```python
from build123d import *

# Parameters (mm, degrees)
ESBO_O1_W                = 4
ESBO_O1_H                = 4
RESSALTO_EXTRUS_O1_DEPTH = 1000
PADR_OCIRCULAR1_COUNT    = 4
FILETE1_R                = 1


with BuildPart() as part:
    # Esboço1 → Ressalto-extrusão1 (new body)
    with BuildSketch(Plane.XY):
        with BuildLine():
            ThreePointArc((-1.664601464, 3.078815026), (-0.858529967, 3.393070335), (0, 3.5))
            Line((0, 3.5), (0, 6))
            Line((0, 6), (-3.878679656, 6))
            Line((-3.878679656, 6), (-8.5, 10.621320344))
            Line((-8.5, 10.621320344), (-8.5, 13))
            Line((-8.5, 13), (-4.1, 13))
            Line((-4.1, 13), (-4.1, 14.5))
            Line((-4.1, 14.5), (-5.1, 14.5))
            Line((-5.1, 14.5), (-5.1, 15))
            Line((-5.1, 15), (-15, 15))
            Line((-15, 15), (-15, 5.1))
            Line((-15, 5.1), (-14.5, 5.1))
            Line((-14.5, 5.1), (-14.5, 4.1))
            Line((-14.5, 4.1), (-13, 4.1))
            Line((-13, 4.1), (-13, 8.5))
            Line((-13, 8.5), (-10.621320344, 8.5))
            Line((-10.621320344, 8.5), (-6, 3.878679656))
            Line((-6, 3.878679656), (-6, 0))
            Line((-6, 0), (-3.5, 0))
            ThreePointArc((-3.5, 0), (-3.393070335, 0.858529967), (-3.078815026, 1.664601464))
            Line((-3.078815026, 1.664601464), (-4.596194078, 3.181980515))
            Line((-4.596194078, 3.181980515), (-3.181980515, 4.596194078))
            Line((-3.181980515, 4.596194078), (-1.664601464, 3.078815026))
        make_face()
        with Locations((-12, 12)):
            Rectangle(ESBO_O1_W, ESBO_O1_H, mode=Mode.SUBTRACT)
    ressalto_extrus_o1 = extrude(amount=RESSALTO_EXTRUS_O1_DEPTH)

    # PadrãoCircular1: Ressalto-extrusão1 ×4 about axis
    padr_ocircular1_axis = Axis((0, 0, 0), (0, 0, 1))
    for i in range(1, PADR_OCIRCULAR1_COUNT):
        add(ressalto_extrus_o1.rotate(padr_ocircular1_axis, i * 360 / PADR_OCIRCULAR1_COUNT))

    # Filete1
    filete1_edges = [part.edges().sort_by_distance(p)[0] for p in [
        (15, -15, 500),
        (15, 15, 500),
        (-15, 15, 500),
        (-15, -15, 500),
    ]]
    fillet(filete1_edges, radius=FILETE1_R)


solid = part.part
```
Source: CAD feature listing. Evaluate the final solid. Frame: model axes, mm. Coordinates: 2 decimals unless noted, no trailing zeros. Put each result on its own line as item: value. Start each with the question number.
1) Ray query, L1, parallel to X at y = -11.75, z = 877; L2, parallel to X at y = 6.25, z = 539. Return the intervals inside material, ascending. Write a range as from..to.
2) Cut plane A-A on z = 291. Give the number of separate pieces and of enclosed holes in the cut face, then the cut area to 3 significant figures.
3) Pull-direction query (Z, two-part tool) for faces 1 (the face through (-1, -4, 0)), 2 (the face through (-1, -4, 1000)); classes: pulls with the +Z half, pulls with the -Z half, needs draft (parallel to the pull), parting line crosses it, or undercut.
4) Contact query for flat-ended pins moving along their axis: pin 1 Ø4 at (y, z) = (2.5, 625.5) entering from -X; pin 2 Ø3 at (x, z) = (2.5, 688.5) entering from -Y; pin 3 Ø4 at (y, z) = (-3, 174) entering from +X. Output: stop coordinate, or through.
The answers:
1. L1: x = -15..-14, -10..-8.5, 8.5..10, 14..15
1. L2: x = -15..-13, -8.37..-4.13, 4.13..8.37, 13..15
2. separate pieces: 1
2. enclosed holes: 5
2. area: 320 mm²
3. face 1: pulls with the -Z half
3. face 2: pulls with the +Z half
4. pin 1: stops at x = -14.5
4. pin 2: stops at y = -6.12
4. pin 3: stops at x = 14.5
